The listing builds one solid part. Answer for the finished solid, in the listing's coordinates (mm). Face numbers are marked on the shaded views. A direction names the side the tool comes from. Round coordinates to 2 decimals unless told otherwise and drop trailing zeros. Order: outer loops, then holes, each group sorted by start corner. A loop starts at its lowest first (then second) coordinate and runs counter-clockwise, first axis right, second up. Notation, with made-up numbers: M 50.5,17.25 L 96.5,17.25 A16 cw 96.5,46.25 Z; hole C 35,29 d10. An arc over 180 degrees is marked long. Write item = value, one per line. Start each with the question number.
(1) A cutting plane is placed at C-C, the plane x = 0.75. Determine the outline of the cut face in (y, z).
(2) Which of the six approach directions +Z, -Z, +X, -X, +Y, -Y give full straight-line access (tool end or side, diameter ignored) to the marked faces 1 and 2?
(3) Each of these flat-tipped pins is pushed along its axis until it touches: pin 1 (4 mm diameter, centred on y = 8, z = -2.5, fed in from -X); pin 2 (3.5 mm diameter, centred on x = 0, z = 0, fed in from -Y); pin 3 (2 mm diameter, centred on y = 10.5, z = 4, fed in from -X). Where does it stop, or does it pass through?
(4) A cutting plane is placed at A-A, the plane z = 0. Determine the outline of the cut face in (x, y).
(5) Straight lines are drawn through the part: probe 1 along Z at (x, y) = (0, 2.25); probe 2 along X at (y, z) = (12.5, 0); probe 3 along Z at (x, y) = (0, 11.25). For each, find the intervals that lie inside material, in ascending order. Write a range as from..to.
(6) A cutting plane is placed at B-B, the plane y = 6.5. Determine the outline of the cut face in (x, z).
(7) For a pull along X with two mould halves and no side action, classify the marked faces 3, 4 and 5 as released by +X, released by -X, zero draft, split by the parting line, or undercut.
(8) A cutting plane is placed at D-D, the plane x = 5.25. Determine the outline of the cut face in (y, z).
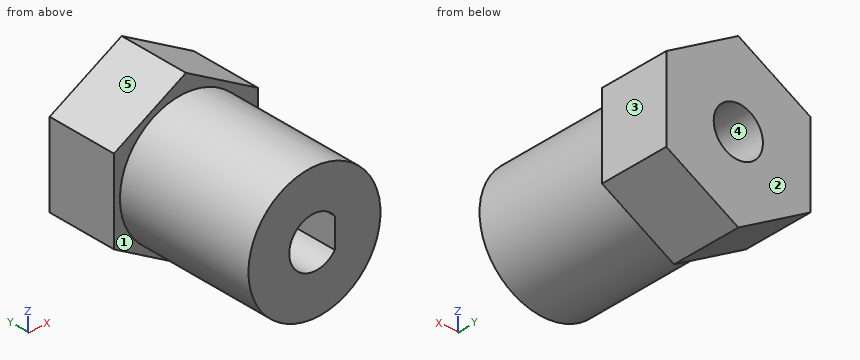
Autodesk Inventor part; units mm, degrees
ref_plane "YZ Plane" through (0, 0, 0) normal (1, 0, 0) x (0, 1, 0)
ref_plane "XZ Plane" through (0, 0, 0) normal (0, 1, 0) x (-1, 0, 0)
ref_plane "XY Plane" through (0, 0, 0) normal (0, 0, 1) x (1, 0, 0)
sketch "草圖1" plane through (0, 0, 0) normal (0, 1, 0) x (-1, 0, 0)
  circle A0 centre (0, 0) radius 5.5
  dimension "d0" = 11
extrude "擠出1" add sketch "草圖1" along normal blind 12
sketch "草圖2" plane through (0, 12, 0) normal (0, 1, 0) x (1, 0, 0)
  line L0 (6, -3.4641) -> (0, -6.9282)
  line L1 (0, -6.9282) -> (-6, -3.4641)
  line L2 (-6, -3.4641) -> (-6, 3.4641)
  line L3 (-6, 3.4641) -> (0, 6.9282)
  line L4 (0, 6.9282) -> (6, 3.4641)
  line L5 (6, 3.4641) -> (6, -3.4641)
  point P0 (0, 0)
  point P1 (0, 0)
  dimension "d3" = 12
extrude "擠出2" add sketch "草圖2" along normal blind 6
sketch "草圖3" plane through (0, 0, 0) normal (0, -1, 0) x (1, 0, 0)
  circle A0 centre (0, 0) radius 2.1
  dimension "d6" = 4.2
extrude "擠出3" cut sketch "草圖3" against normal up to surface (18 mm away)
sketch "草圖5" plane through (0, 0, 0) normal (1, 0, 0) x (0, 1, 0)
  circle A0 centre (4, 0) radius 1.361
  point P0 (0, 0)
  dimension "d12" = 4
extrude "擠出5" [suppressed]
sketch "草圖7" plane through (0, 0, 0) normal (0, -1, 0) x (1, 0, 0)
  circle A0 centre (0, 0) radius 2.1
  line L0 (1.7, -1.2329) -> (1.7, 1.2329)
  dimension "d16" = 1.7
extrude "擠出6" add sketch "草圖7" against normal blind 8 contours A0 L0 picked at (1.773, -0.2844)
sketch "草圖8" plane through (0, 18, 0) normal (0, 1, 0) x (1, 0, 0)
  circle A0 centre (0, 0) radius 2.05
  circle A1 centre (0, 0) radius 2.1
  dimension "d19" = 4.1
extrude "擠出7" add sketch "草圖8" against normal up to surface (10 mm away)
properties part number "Coupling_print"
Reported:
q1.outline = M 0,-5.45 L 12,-5.45 L 12,-6.5 L 18,-6.5 L 18,-1.91 L 8,-1.91 L 8,-1.96 L 0,-1.96 Z; M 0,1.96 L 8,1.96 L 8,1.91 L 18,1.91 L 18,6.5 L 12,6.5 L 12,5.45 L 0,5.45 Z
q2.face_1 = -Y
q2.face_2 = +Z, -Z, +X, -X, +Y
q3.pin_1 = -5.48
q3.pin_2 = 0
q3.pin_3 = -4.61
q4.outline = M -6,12 L -5.5,12 L -5.5,0 L -2.1,0 L -2.1,8 L -2.05,8 L -2.05,18 L -6,18 Z; M 1.7,0 L 5.5,0 L 5.5,12 L 6,12 L 6,18 L 2.05,18 L 2.05,8 L 1.7,8 Z
q5.probe_1 = -5.5..-2.1, 2.1..5.5
q5.probe_2 = -6..-2.05, 2.05..6
q5.probe_3 = -5.5..-2.05, 2.05..5.5
q6.outline = C 0,0 d11; hole M 1.7,-1.23 L 1.7,1.23 A2.1 ccw long Z
q7.face_3 = released by +X
q7.face_4 = undercut
q7.face_5 = released by -X
q8.outline = M 0,-1.64 L 12,-1.64 L 12,-3.9 L 18,-3.9 L 18,3.9 L 12,3.9 L 12,1.64 L 0,1.64 Z
